Autodesk Inventor part; units mm, degrees
ref_plane "YZ Plane" through (0, 0, 0) normal (1, 0, 0) x (0, 1, 0)
ref_plane "XZ Plane" through (0, 0, 0) normal (0, 1, 0) x (-1, 0, 0)
ref_plane "XY Plane" through (0, 0, 0) normal (0, 0, 1) x (1, 0, 0)
sketch "Sketch1" plane through (0, 0, 0) normal (0, 0, 1) x (1, 0, 0)
  line L0 (-13.5, 15) -> (13.5, 15)
  line L1 (15.5, 13) -> (15.5, -13)
  line L2 (13.5, -15) -> (-13.5, -15)
  line L3 (-15.5, -13) -> (-15.5, 13)
  line L4 (-22.2799, 0) -> (22.2799, 0)
  line L5 (0, -21.5799) -> (0, 21.5799)
  circle A0 centre (-12, 12) radius 1.5
  arc A1 (-13.5, 15) -> (-15.5, 13) centre (-13.5, 13) ccw
  arc A2 (15.5, 13) -> (13.5, 15) centre (13.5, 13) ccw
  arc A3 (13.5, -15) -> (15.5, -13) centre (13.5, -13) ccw
  arc A4 (-15.5, -13) -> (-13.5, -15) centre (-13.5, -13) ccw
  circle A5 centre (12, 12) radius 1.5
  circle A6 centre (-12, -12) radius 1.5
  circle A7 centre (12, -12) radius 1.5
  point P0 (0, 0)
  point P1 (-15.5, 15)
  point P2 (15.5, -15)
  point P3 (15.5, 15)
  point P4 (13.5, 13)
  dimension "d0" = 31
  dimension "d1" = 30
  dimension "d2" = 15
  dimension "d3" = 15.5
  dimension "d4" = 3
  dimension "d5" = 12
  dimension "d6" = 12
  dimension "d7" = 2
extrude "Extrusion1" add sketch "Sketch1" along normal blind 0.9
sketch "Sketch2" plane through (0, 0, 0.9) normal (0, 0, 1) x (1, 0, 0)
  circle A0 centre (12, -12) radius 1.5
  circle A1 centre (-12, -12) radius 1.5
  circle A2 centre (12, 12) radius 1.5
  circle A3 centre (-12, 12) radius 1.5
  line L0 (13.5, 15) -> (-13.5, 15)
  arc A4 (-13.5, 15) -> (-15.5, 13) centre (-13.5, 13) ccw
  line L1 (-15.5, 13) -> (-15.5, -13)
  arc A5 (-15.5, -13) -> (-13.5, -15) centre (-13.5, -13) ccw
  line L2 (-13.5, -15) -> (13.5, -15)
  arc A6 (13.5, -15) -> (15.5, -13) centre (13.5, -13) ccw
  line L3 (15.5, -13) -> (15.5, 13)
  arc A7 (15.5, 13) -> (13.5, 15) centre (13.5, 13) ccw
  line L4 (-15.5, 12) -> (-14.6, 12)
  line L5 (-14.6, 12) -> (-14.6, -12)
  line L6 (-14.6, -12) -> (-15.5, -12)
  line L7 (-15.5, -12) -> (-15.5, 12)
  line L8 (-22.2799, 0) -> (22.2799, 0)
  line L9 (0, -21.5799) -> (0, 21.5799)
  point P0 (0, 0)
  dimension "d10" = 0.9
  dimension "d11" = 24
  dimension "d12" = 12
extrude "Extrusion2" add sketch "Sketch2" along normal blind 26.1 contours L8 L1 L4 L5 | L5 L6 L1 L8
fillet "Fillet1" radius 1 1 edges at (-14.6, 0, 0.9)
sketch "Sketch3" plane through (-14.6, -12, 27) normal (1, 0, 0) x (0, 0, -1)
  line L0 (27, -1) -> (27, 25)
  line L1 (27, -1) -> (26.1, -1)
  line L2 (26.1, 0) -> (26.1, -1)
  line L3 (26.1, 0) -> (0, 0)
  line L4 (0, 24) -> (0, 0)
  line L5 (26.1, 24) -> (0, 24)
  line L6 (26.1, 25) -> (26.1, 24)
  line L7 (27, 25) -> (26.1, 25)
  line L8 (35.3744, 12) -> (2.9643, 12) construction
  circle A0 centre (12, 12) radius 12
  point P0 (27, 12)
  dimension "d16" = 15
  dimension "d17" = 24
extrude "Extrusion3" add sketch "Sketch3" along normal blind 30.1 contours A0
sketch "Sketch4" plane through (-15.5, -13, 0) normal (-1, 0, 0) x (0, 0, 1)
  circle A0 centre (15, 13) radius 12
  arc A1 (15, 25) -> (15, 1) centre (15, 13) ccw
  arc A2 (27, 13) -> (15, 25) centre (15, 13) ccw
  arc A3 (15, 1) -> (27, 13) centre (15, 13) ccw
  circle A4 centre (15, 13) radius 12.5
  point P0 (0, 13)
  dimension "d20" = 25
extrude "Extrusion4" add sketch "Sketch4" along normal blind 16.5 contours A0 | A4
sketch "Sketch5" plane through (15.5, 0, 15) normal (1, 0, 0) x (0, 0, -1)
  circle A0 centre (0, 0) radius 12
  arc A1 (0, -12) -> (0, 12) centre (0, 0) ccw
  arc A2 (0, 12) -> (-12, 0) centre (0, 0) ccw
  arc A3 (-12, 0) -> (0, -12) centre (0, 0) ccw
  circle A4 centre (0, 0) radius 4.25
  point P0 (15, 0)
  dimension "d23" = 8.5
extrude "Extrusion5" add sketch "Sketch5" along normal blind 2 contours A4
sketch "Sketch6" plane through (15.5, 0, 15) normal (1, 0, 0) x (0, 0, -1)
  circle A0 centre (0, 0) radius 12
  arc A1 (0, -12) -> (0, 12) centre (0, 0) ccw
  arc A2 (0, 12) -> (-12, 0) centre (0, 0) ccw
  arc A3 (-12, 0) -> (0, -12) centre (0, 0) ccw
  line L0 (0, 12.481) -> (0, -10.3275) construction
  line L1 (-1, -9.75) -> (1, -9.75)
  line L2 (1, -9.75) -> (1, -9.25)
  line L3 (1, -9.25) -> (-1, -9.25)
  line L4 (-1, -9.25) -> (-1, -9.75)
  line L5 (0, 0) -> (-4.6495, 0) construction
  line L6 (-1, 9.75) -> (1, 9.75)
  line L7 (1, 9.75) -> (1, 9.25)
  line L8 (1, 9.25) -> (-1, 9.25)
  line L9 (-1, 9.25) -> (-1, 9.75)
  point P0 (15, 0)
  point P1 (0, 10.3275)
  dimension "d26" = 2
  dimension "d27" = 1
  dimension "d28" = 0.5
  dimension "d29" = 9.25
extrude "Extrusion6" add sketch "Sketch6" along normal blind 4 contours L4 L3 L2 L1 | L6 L7 L8 L9
sketch "Sketch7" plane through (15.5, -9.75, 14) normal (0, -1, 0) x (1, 0, 0)
  line L0 (0, 0) -> (0, 2)
  line L1 (0, 0) -> (4, 0)
  line L2 (4, 2) -> (4, 0)
  line L3 (0, 2) -> (4, 2)
  line L4 (4, 1) -> (0, 1) construction
  line L5 (0, 0) -> (0, 2)
  circle A0 centre (2.95, 1) radius 0.75
  point P0 (-15.5, -14)
  dimension "d32" = 1.5
  dimension "d33" = 1.05
extrude "Extrusion7" cut sketch "Sketch7" against normal through all contours A0
fillet "Fillet2" radius 1 2 edges at (19.5, -9.5, 16) (19.5, -9.5, 14)
fillet "Fillet3" radius 1 2 edges at (19.5, 9.5, 16) (19.5, 9.5, 14)
sketch "Sketch8" plane through (-32, 0, 15) normal (-1, 0, 0) x (0, 0, 1)
  circle A0 centre (0, 0) radius 12.5
  circle A1 centre (0, 0) radius 2.485
  point P0 (-15, 0)
  dimension "d38" = 4.97
extrude "Extrusion8" add sketch "Sketch8" along normal blind 6 contours A1
sketch "Sketch9" plane through (-38, 0, 15) normal (-1, 0, 0) x (0, 0, 1)
  circle A0 centre (0, 0) radius 2.485
  circle A1 centre (0, 0) radius 0.99
  point P0 (-15, 0)
  dimension "d41" = 1.98
extrude "Extrusion9" add sketch "Sketch9" along normal blind 6.5 contours A1
sketch "Sketch10" plane through (0, 0, 0) normal (0, 1, 0) x (-1, 0, 0)
  line L0 (44.5, 14.01) -> (44.5, 15.99)
  line L1 (38, 15.99) -> (38, 14.01)
  line L2 (42, 15.99) -> (39, 15.99)
  line L3 (39, 15.99) -> (39, 15.49)
  line L4 (39, 15.49) -> (42, 15.49)
  line L5 (42, 15.49) -> (42, 15.99)
  line L6 (38, 15.99) -> (44.5, 15.99) construction
  line L7 (38, 15.99) -> (44.5, 15.99)
  point P0 (0, 0)
  dimension "d44" = 3
  dimension "d45" = 0.5
  dimension "d46" = 1
extrude "Extrusion10" cut sketch "Sketch10" along normal mid plane 6.5
equation "\"d2\" = 0.5 * d1"
equation "\"d3\" = 0.5 * d0"
equation "\"d12\" = 0.5 * d11"
equation "\"d27\" = 0.5 * d26"
properties part number "BallBallancing_DCmotor"
Verification items for the finished model (mm, model axes). A direction names the side the tool comes from. Give positions to 0.01 mm unless a question says otherwise; leave off trailing zeros. Order: outer loops, then holes, each group sorted by start corner. A loop starts at its lowest first (then second) coordinate and runs counter-clockwise, first axis right, second up. Notation, with made-up numbers: (8, -5.75) -> (64, -5.75) arc R12 cw to (64, 0.25) -> close; hole circle Ø2 at (32.25, -4.75). An arc over 180 degrees is marked (long way). Use a Markdown table: item, result.
1) Material ranges on probe 1 along Z at (x, y) = (18.45, 9.55); probe 2 along Y at (x, z) = (12, 0.65); probe 3 along X at (y, z) = (-9, 13), recorded low to high.
Results:
| item | result |
|---|---|
| probe 1 | 14 to 14.25, 15.75 to 16 |
| probe 2 | -15 to -13.5, -10.5 to 10.5, 13.5 to 15 |
| probe 3 | -32 to 15.5 |
2) Mould release check, pull along Z, two halves, no side actions. Record for faces 5 (the flat face through (-14.6, 0.1, 2.6)), 6 (the cylindrical face through (-34.96, -0.75, 17.37)), 7 (the cylindrical face through (-13.5, 11.93, 0.44)): pulls with the +Z half, pulls with the -Z half, needs draft (parallel to the pull), parting line crosses it, or undercut.
Results:
| item | result |
|---|---|
| face 5 | undercut |
| face 6 | parting line crosses it |
| face 7 | needs draft |
3) Section check B-B, the plane x = -2.5. Record the boundary of the cut face in (y, z), then the cut area to 3 significant figures.
Results:
| item | result |
|---|---|
| outline | (-15, 0) -> (15, 0) -> (15, 0.9) -> (-15, 0.9) -> close; circle Ø24 at (0, 15) |
| area | 479 mm² |
4) Tool access check on faces 1 (the flat face through (-15.5, -10, 25)), 2 (the cylindrical face through (10.5, 11.93, 0.44)), 3 (the flat face through (-38, -1, 16)), 4 (the flat face through (-15, -12, 14)). Record the directions out of +Z, -Z, +X, -X, +Y, -Y that give a thin tool (end or side, any length) a straight path to the whole face; none if there is none.
Results:
| item | result |
|---|---|
| face 1 | +Z, -X, -Y |
| face 2 | -Z |
| face 3 | -X |
| face 4 | +Z, +X, -Y |
5) Section check A-A, the plane x = 12. Record the boundary of the cut face in (y, z), then the cut area to 3 significant figures.
Results:
| item | result |
|---|---|
| outline | (-15, 0) -> (-13.5, 0) -> (-13.5, 0.9) -> (-15, 0.9) -> close; circle Ø24 at (0, 15); (-10.5, 0) -> (10.5, 0) -> (10.5, 0.9) -> (-10.5, 0.9) -> close; (13.5, 0) -> (15, 0) -> (15, 0.9) -> (13.5, 0.9) -> close |
| area | 474 mm² |
6) Section check D-D, the plane z = 24. Record the boundary of the cut face in (x, y).
Results:
| item | result |
|---|---|
| outline | (-32, -8.67) -> (-15.5, -8.67) -> (-15.5, -12) -> (-14.6, -12) -> (-14.6, -7.94) -> (15.5, -7.94) -> (15.5, 7.94) -> (-14.6, 7.94) -> (-14.6, 12) -> (-15.5, 12) -> (-15.5, 8.67) -> (-32, 8.67) -> close |
7) Section check C-C, the plane y = 1.75. Record the boundary of the cut face in (x, z), then the cut area to 3 significant figures.
Results:
| item | result |
|---|---|
| outline | (-38, 13.24) -> (-32, 13.24) -> (-32, 2.62) -> (-15.5, 2.62) -> (-15.5, 0) -> (15.5, 0) -> (15.5, 0.9) -> (-13.6, 0.9) arc R1 cw to (-14.6, 1.9) -> (-14.6, 3.13) -> (15.5, 3.13) -> (15.5, 11.13) -> (17.5, 11.13) -> (17.5, 18.87) -> (15.5, 18.87) -> (15.5, 26.87) -> (-14.6, 26.87) -> (-14.6, 27) -> (-15.5, 27) -> (-15.5, 27.38) -> (-32, 27.38) -> (-32, 16.76) -> (-38, 16.76) -> close |
| area | 1,210 mm² |
8) Depth check by flat-ended pin: pin 1 Ø1.4 at (x, y) = (-41, 0) entering from +Z; pin 2 Ø1 at (x, z) = (-5, 11) entering from +Y; pin 3 Ø1 at (x, y) = (-32, 9) entering from +Z. Enter the tip coordinate at first touch or a pass-through.
Results:
| item | result |
|---|---|
| pin 1 | z = 15.49 |
| pin 2 | y = 11.48 |
| pin 3 | z = 24.17 |
